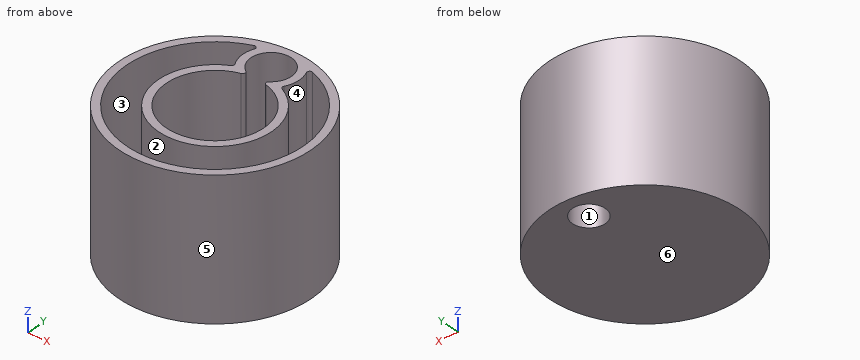
```python
from build123d import *

# Parameters (mm, degrees)
F0_R     = 18.542
F0_R_2   = 3.175
F1_DEPTH = 7.62
F2_R     = 18.542
F3_DEPTH = 19.05
F4_R     = 0.508


with BuildPart() as f1:
    # F0 (on Top) → F1 (new body)
    with BuildSketch(Plane.XY):
        Circle(F0_R)
        with Locations((0, 13.208)):
            Circle(F0_R_2, mode=Mode.SUBTRACT)
    extrude(amount=F1_DEPTH)

    # F2 (on face) → F3 (join)
    with BuildSketch(Plane.XY.offset(7.62)):
        Circle(F2_R)
        with BuildLine():
            ThreePointArc((-4.3636460762, 16.44904), (-5.435558049, 13.2293554581), (-4.3889780516, 10.0013476923))
            ThreePointArc((-4.3889780516, 10.0013476923), (0, -10.922), (4.3889780516, 10.0013476923))
            ThreePointArc((4.3889780516, 10.0013476923), (5.435558049, 13.2293554581), (4.3636460762, 16.44904))
            ThreePointArc((4.3636460762, 16.44904), (0, -17.018), (-4.3636460762, 16.44904))
        make_face(mode=Mode.SUBTRACT)
        with BuildLine():
            ThreePointArc((-0.7465455676, 9.3683015385), (0, 17.1196), (0.7465455676, 9.3683015385))
            ThreePointArc((0.7465455676, 9.3683015385), (0, -9.398), (-0.7465455676, 9.3683015385))
        make_face(mode=Mode.SUBTRACT)
    extrude(amount=F3_DEPTH)

    # F4
    f4_edges = [f1.edges().sort_by_distance(p)[0] for p in [
        (0.746546, 9.368302, 17.145),
        (4.388978, 10.001348, 17.145),
        (4.363646, 16.44904, 17.145),
        (-4.388978, 10.001348, 17.145),
        (-4.363646, 16.44904, 17.145),
        (-0.746546, 9.368302, 17.145),
    ]]
    fillet(f4_edges, radius=F4_R)


solid = f1.part
```
Design review of the part built by this model. Coordinates are the model's own, in mm. Face numbers are marked on the shaded views. A direction names the side the tool comes from. Coordinates: 2 decimals unless noted, no trailing zeros. Loops run counter-clockwise (first coordinate to the right, second up) from the corner with the lowest first, then second, coordinate; pieces in that order, holes last.
Q1. We need section C-C on y = 12.5. State the section outline as (x, z) points.
Reported:
outline: (-13.7, 0) - (-3.1, 0) - (-3.1, 7.62) - (-3.85, 7.62) - (-3.85, 26.67) - (-5.39, 26.67) - (-5.39, 7.62) - (-11.55, 7.62) - (-11.55, 26.67) - (-13.7, 26.67) - close; (3.1, 0) - (13.7, 0) - (13.7, 26.67) - (11.55, 26.67) - (11.55, 7.62) - (5.39, 7.62) - (5.39, 26.67) - (3.85, 26.67) - (3.85, 7.62) - (3.1, 7.62) - close
Q2. We need section A-A on x = 0. State the section outline as (y, z) points, and give its area (3 significant figures).
Reported:
outline: (-18.54, 0) - (10.03, 0) - (10.03, 7.62) - (-9.4, 7.62) - (-9.4, 26.67) - (-10.92, 26.67) - (-10.92, 7.62) - (-17.02, 7.62) - (-17.02, 26.67) - (-18.54, 26.67) - close; (16.38, 0) - (18.54, 0) - (18.54, 26.67) - (17.12, 26.67) - (17.12, 7.62) - (16.38, 7.62) - close
area: 319 mm2
Q3. The part is to be moulded in two halves that separate along X. For the marked faces 3, 4, 5 and 6, say which applies: +X half, -X half, draft (parallel to the pull), parting line (faces both ways), or undercut.
Reported:
face 3: undercut
face 4: undercut
face 5: parting line
face 6: draft
Q4. For pin 1 (2 mm diameter, centred on x = -0.5, y = 7, fed in from +Z); pin 2 (5 mm diameter, centred on y = -6, z = 4, fed in from -X); pin 3 (2 mm diameter, centred on x = 5.5, z = 18.5, fed in from -Y), all flat-tipped, find the tip position at first contact; note any pin that passes through.
Reported:
pin 1: stops at z = 7.62
pin 2: stops at x = -18.21
pin 3: stops at y = -17.99
Q5. We need section B-B on y = 0. State the section outline as (x, z) points, and give its area (3 significant figures).
Reported:
outline: (-18.54, 0) - (18.54, 0) - (18.54, 26.67) - (17.02, 26.67) - (17.02, 7.62) - (10.92, 7.62) - (10.92, 26.67) - (9.4, 26.67) - (9.4, 7.62) - (-9.4, 7.62) - (-9.4, 26.67) - (-10.92, 26.67) - (-10.92, 7.62) - (-17.02, 7.62) - (-17.02, 26.67) - (-18.54, 26.67) - close
area: 399 mm2
Q6. We need section D-D on x = -12.5. State the section outline as (y, z) points.
Reported:
outline: (-13.7, 0) - (13.7, 0) - (13.7, 26.67) - (11.55, 26.67) - (11.55, 7.62) - (-11.55, 7.62) - (-11.55, 26.67) - (-13.7, 26.67) - close
Q7. To check wall thickness, follow line 1 (Y direction, x = 0, z = 13.5); line 2 (X direction, y = 4, z = 20.5); line 3 (X direction, y = 1, z = 21). State the ranges of each line that lie inside material, in increasing order.
Reported:
line 1: y = -18.54 to -17.02, -10.92 to -9.4, 17.12 to 18.54
line 2: x = -18.11 to -16.54, -10.16 to -8.5, 8.5 to 10.16, 16.54 to 18.11
line 3: x = -18.52 to -16.99, -10.88 to -9.34, 9.34 to 10.88, 16.99 to 18.52
Q8. Tool access review of the marked faces 1 and 2: name each direction out of +Z, -Z, +X, -X, +Y, -Y from which nothing blocks a thin tool from reaching the whole face with its end or side.
Reported:
face 1: +Z, -Z
face 2: +Z
